Source: CAD feature listing. Evaluate the final solid. Frame: model axes, mm. A direction names the side the tool comes from. Give positions to 0.01 mm unless a question says otherwise; leave off trailing zeros. Loops run counter-clockwise (first coordinate to the right, second up) from the corner with the lowest first, then second, coordinate; pieces in that order, holes last. Notation, with made-up numbers: (69, 51.5) - (128, 51.5) arc R28 cw to (128, 86.5) - close; hole circle Ø5 at (49.5, 68). An arc over 180 degrees is marked (long way). Put each result on its own line as item: value.
```python
from build123d import *

# Parameters (mm, degrees)
ESBO_O2_W = 6.7
ESBO_O2_H = 8.7


with BuildPart() as part:
    # Esboço2 → Revolução1 (revolve)
    with BuildSketch(Plane.XY):
        with Locations((-3.35, 49.55)):
            Rectangle(ESBO_O2_W, ESBO_O2_H)
        Polygon((-3.65, 44.2), (-3.65, 26.95), (0, 26.95), (0, 45.2), (-3.65, 45.2), align=None)
        Polygon((-3.65, 26.95), (-3.65, 9.7), (-3.65, 8.7), (0, 8.7), (0, 26.95), align=None)
        with Locations((-3.35, 4.35)):
            Rectangle(ESBO_O2_W, ESBO_O2_H)
        Polygon((-3.65, 9.7), (-6.7, 8.7), (-3.65, 8.7), align=None)
        Polygon((-6.7, 45.2), (-3.65, 44.2), (-3.65, 45.2), align=None)
    revolve(axis=Axis((0, -28.709318564, 0), (0, 1, 0)))


solid = part.part
```
1) Pin query (flat end, axial travel): P1, Ø2, axis at x = -3, y = 22.5, coming from the +Z side; P2, Ø3, axis at x = -3.5, z = 1, coming from the -Y side; P3, Ø6, axis at y = 23.5, z = -1, coming from the -X side; P4, Ø4, axis at x = 3, y = 15.5, coming from the -Z side. Return the tip coordinate at first contact, or that it passes through.
Check result:
P1: z = 3.05
P2: y = 0
P3: x = -3.65
P4: z = -3.51
2) Section query A-A, the plane z = 0. Output: boundary loops of the cut face in (x, y), plus the area to 3 significant figures.
Check result:
outline: (-6.7, 0) - (6.7, 0) - (6.7, 8.7) - (3.65, 9.7) - (3.65, 44.2) - (6.7, 45.2) - (6.7, 53.9) - (-6.7, 53.9) - (-6.7, 45.2) - (-3.65, 44.2) - (-3.65, 9.7) - (-6.7, 8.7) - close
area: 506 mm²
3) Mould query, pull axis Y, two halves, no side actions, for faces 3 (the flat face through (0, 53.9, 0)), 4 (the conical face through (0.82, 44.25, -3.71)), 5 (the flat face through (0, 0, 0)), 6 (the cylindrical face through (6.694, 49.611, 0.295)). Classes: pulls with the +Y half, pulls with the -Y half, needs draft (parallel to the pull), parting line crosses it, or undercut.
Check result:
face 3: pulls with the +Y half
face 4: undercut
face 5: pulls with the -Y half
face 6: needs draft
4) Access query for faces 1 (the cylindrical face through (6.694, 4.411, 0.295)), 2 (the cylindrical face through (-3.48, 26.71, 1.1)). Directions: +Z, -Z, +X, -X, +Y, -Y. A direction counts if a zero-diameter tool reaches every point of the face in a straight line with its end or side. Return the directions, or none.
Check result:
face 1: +Y, -Y
face 2: none
5) Material intervals for line 1 along Y through (x, z) = (-4, 3.5); line 2 along Y through (x, z) = (1.5, -4.25); line 3 along X through (y, z) = (31.5, 2), sorted ascending. Write a range as [from, to].
Check result:
line 1: [0, 9.15], [44.75, 53.9]
line 2: [0, 9.42], [44.48, 53.9]
line 3: [-3.05, 3.05]
6) Section query C-C, the plane y = 36. Output: boundary loops of the cut face in (x, z), plus the area to 3 significant figures.
Check result:
outline: circle Ø7.3 at (0, 0)
area: 41.9 mm²
7) Section query B-B, the plane x = 0. Output: boundary loops of the cut face in (y, z).
Check result:
outline: (0, -6.7) - (8.7, -6.7) - (9.7, -3.65) - (44.2, -3.65) - (45.2, -6.7) - (53.9, -6.7) - (53.9, 6.7) - (45.2, 6.7) - (44.2, 3.65) - (9.7, 3.65) - (8.7, 6.7) - (0, 6.7) - close
